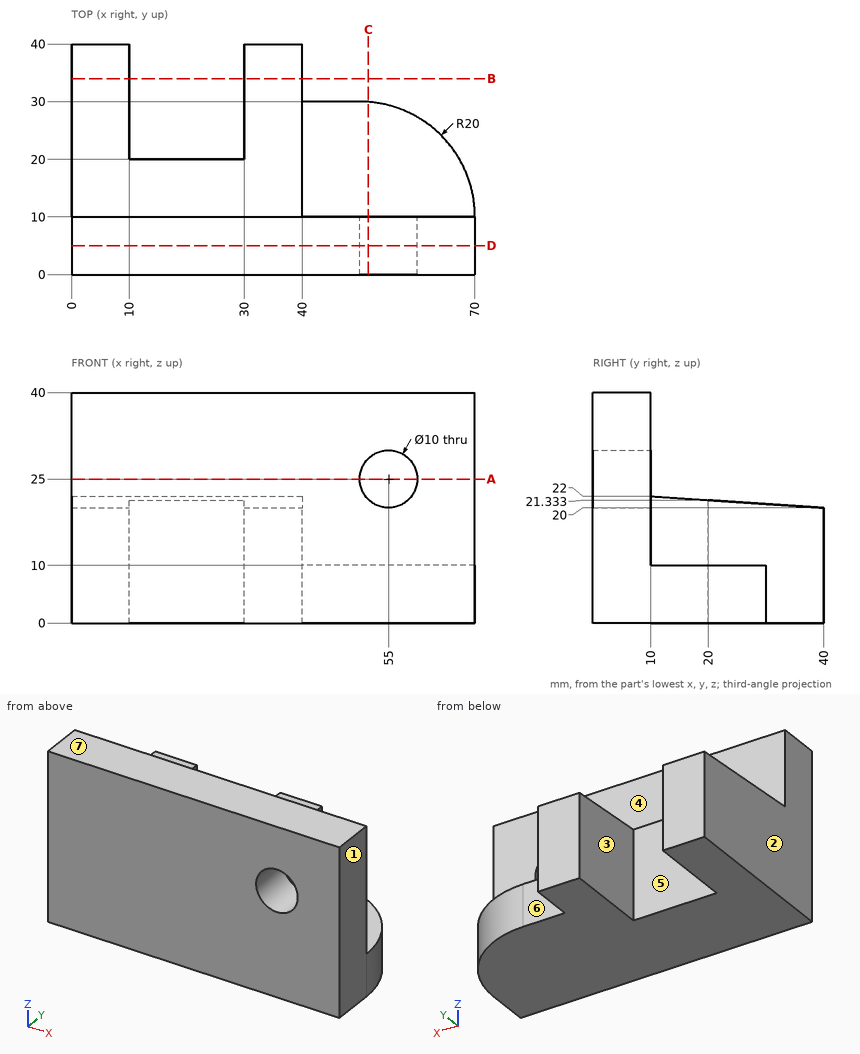
Answer from the drawing. Dimensions are ordinates in mm from the lowest x, y and z of the part. A direction names the side the tool comes from. Round coordinates to 2 decimals unless told otherwise and drop trailing zeros. Write each loop counter-clockwise with the first axis right and the second up, starting at its lowest first coordinate (ties: lowest second). Pieces come first, ordered by that corner, then holes. Notation, with made-up numbers: (3.5, -24) - (41.5, -24) arc R25 ccw to (41.5, 4) - close; hole circle Ø1 at (-8.5, -35). An arc over 180 degrees is marked (long way). One line per item, written item: value.
Q1. Find section D-D (y = 5). Determine the outline of the cut face in (x, z), and give its area (3 significant figures).
The answers:
outline: (0, 0) - (70, 0) - (70, 40) - (0, 40) - close; hole circle Ø10 at (55, 25)
area: 2,720 mm2
Q2. Which of the six approach directions +Z, -Z, +X, -X, +Y, -Y give full straight-line access (tool end or side, diameter ignored) to the marked faces 5, 6 and 7?
The answers:
face 5: +Z, -Z, +Y
face 6: +Z, -Z, +X, +Y
face 7: +Z, +X, -X, +Y, -Y
Q3. Find section B-B (y = 34). Determine the outline of the cut face in (x, z).
The answers:
outline: (0, 0) - (10, 0) - (10, 20.4) - (0, 20.4) - close; (30, 0) - (40, 0) - (40, 20.4) - (30, 20.4) - close
Q4. Find section C-C (x = 51.5). Determine the outline of the cut face in (y, z).
The answers:
outline: (0, 0) - (29.94, 0) - (29.94, 10) - (10, 10) - (10, 21.43) - (0, 21.43) - close; (0, 28.57) - (10, 28.57) - (10, 40) - (0, 40) - close
Q5. Straight lines are drawn through the part: line 1 (X direction, y = 4, z = 25); line 2 (X direction, y = 21.5, z = 14); line 3 (Z direction, x = 55, y = 4). For each, find the intervals that lie inside material, in ascending order. Write a range as from..to.
The answers:
line 1: x = 0..50, 60..70
line 2: x = 0..10, 30..40
line 3: z = 0..20, 30..40
Q6. Each of these flat-tipped pins is pushed along its axis until it touches: P1, Ø17.5, axis at y = 20, z = 13, coming from the +X side; P2, Ø6, axis at x = 21, z = 7.5, coming from the +Y side; P3, Ø24, axis at x = 27.5, z = 24.5, coming from the +Y side; P4, Ø5, axis at x = 11.5, y = 30, coming from the +Z side. Where does it stop, or does it pass through?
The answers:
P1: stops at x = 69.92
P2: stops at y = 20
P3: stops at y = 40
P4: stops at z = 20.8
Q7. Find section A-A (z = 25). Determine the outline of the cut face in (x, y), and give its area (3 significant figures).
The answers:
outline: (0, 0) - (50, 0) - (50, 10) - (0, 10) - close; (60, 0) - (70, 0) - (70, 10) - (60, 10) - close
area: 600 mm2
Q8. For a pull along X with two mould halves and no side action, classify the marked faces 1, 2, 3 and 4 as pulls with the +X half, pulls with the -X half, needs draft (parallel to the pull), parting line crosses it, or undercut.
The answers:
face 1: pulls with the +X half
face 2: pulls with the -X half
face 3: undercut
face 4: needs draft
